```python
from build123d import *

# Parameters (mm, degrees)
SKETCH1_R               = 20.35
BOSS_EXTRUDE2_DEPTH     = 5
SKETCH1_3_R             = 2.35
BOSS_EXTRUDE3_DEPTH     = 10
SKETCH2_R               = 14.85
BOSS_EXTRUDE4_DEPTH     = 7
SKETCH3_R               = 6
SKETCH3_R_2             = 4.1
BOSS_EXTRUDE5_DEPTH     = 10
CUT_EXTRUDE1_DEPTH      = 34.425215033
CUT_EXTRUDE1_DEPTH_BACK = 34.425215033
SKETCH5_R               = 1.6
SKETCH6_R               = 10
CUT_EXTRUDE2_DEPTH      = 9


with BuildPart() as part:
    # Sketch1 → Boss-Extrude2 (new body)
    with BuildSketch(Plane(origin=(0, 0, 0), x_dir=(1, 0, 0), z_dir=(0, 1, 0))):
        with Locations(Location((0, 0, 0), (0, 0, 270))):
            Circle(SKETCH1_R)
    extrude(amount=BOSS_EXTRUDE2_DEPTH)

    # Sketch1_3 → Boss-Extrude3 (add)
    with BuildSketch(Plane(origin=(0, 0, 0), x_dir=(1, 0, 0), z_dir=(0, 1, 0))):
        with Locations(Location((0, 18, 0), (0, 0, 89.999437987))):
            Circle(SKETCH1_3_R)
        with Locations(Location((-17.119017293, 5.562305899, 0), (0, 0, 161.999437549))):
            Circle(SKETCH1_3_R)
        with Locations(Location((-10.580134541, -14.562305899, 0), (0, 0, 233.999434816))):
            Circle(SKETCH1_3_R)
        with Locations(Location((10.580134541, -14.562305899, 0), (0, 0, 305.999433126))):
            Circle(SKETCH1_3_R)
        with Locations(Location((17.119017293, 5.562305899, 0), (0, 0, 17.99943498))):
            Circle(SKETCH1_3_R)
    extrude(amount=BOSS_EXTRUDE3_DEPTH)

    # Sketch2 → Boss-Extrude4 (add)
    with BuildSketch(Plane.XZ):
        with Locations(Location((0, 0, 0), (0, 0, 270))):
            Circle(SKETCH2_R)
    extrude(amount=BOSS_EXTRUDE4_DEPTH)

    # Sketch3 → Boss-Extrude5 (add)
    with BuildSketch(Plane.XZ.offset(7)):
        with Locations(Location((0, 0, 0), (0, 0, 270))):
            Circle(SKETCH3_R)
        with Locations(Location((0, 0, 0), (0, 0, 270))):
            Circle(SKETCH3_R_2, mode=Mode.SUBTRACT)
    extrude(amount=BOSS_EXTRUDE5_DEPTH)

    # Sketch5 → Cut-Extrude1 (cut, two sides: drawn at the far end of the back side and taken through both)
    with BuildSketch(Plane(origin=(0, 0, 0), x_dir=(0, 0, -1), z_dir=(1, 0, 0)).offset(-CUT_EXTRUDE1_DEPTH_BACK)):
        with Locations((0, -11.941738225)):
            Circle(SKETCH5_R)
    extrude(amount=CUT_EXTRUDE1_DEPTH + CUT_EXTRUDE1_DEPTH_BACK, mode=Mode.SUBTRACT)

    # Sketch6 → Cut-Extrude2 (cut)
    with BuildSketch(Plane(origin=(0, 5, 0), x_dir=(1, 0, 0), z_dir=(0, 1, 0))):
        with Locations(Location((0, 0, 0), (0, 0, 270))):
            Circle(SKETCH6_R)
    extrude(amount=-CUT_EXTRUDE2_DEPTH, mode=Mode.SUBTRACT)


solid = part.part
```
The listing builds one solid part. Answer for the finished solid, in the listing's coordinates (mm). A direction names the side the tool comes from. Round coordinates to 2 decimals unless told otherwise and drop trailing zeros. Order: outer loops, then holes, each group sorted by start corner. A loop starts at its lowest first (then second) coordinate and runs counter-clockwise, first axis right, second up. Notation, with made-up numbers: (18.25, 16.5) -> (43.25, 16.5) arc R22 cw to (43.25, 30.5) -> close; hole circle Ø2 at (65.5, 13.5). An arc over 180 degrees is marked (long way). Answer as CSV lines item,"result". Start each with the question number.
(1) The part is cut by section C-C (z = -13). Determine the outline of the cut face in (x, y), then the cut area to 3 significant figures.
(2) Find the intervals of material crossed by probe 1 along X at (y, z) = (-2, 0); probe 2 along Y at (x, z) = (5, 0); probe 3 along X at (y, z) = (0.75, 0), in increasing order. Write a range as from..to.
(3) For a pull along Z with two mould halves and no side action, classify faces 1 (the face through (-9.04, -3.45, 11.78)), 2 (the face through (-4, -17, -3)), 3 (the face through (1.23, -11.93, -3.91)) as +Z half, -Z half, draft (parallel to the pull), parting line (faces both ways), or undercut.
(4) The part is cut by section B-B (y = -9.75). Determine the outline of the cut face in (x, z), then the cut area to 3 significant figures.
(5) The part is cut by section A-A (z = 0). Determine the outline of the cut face in (x, y), then the cut area to 3 significant figures.
(6) A tool of negligible diameter and unlimited length cuts with its end or side. For faces 4 (the face through (-9.72, 7.46, 16.75)), 5 (the face through (-6.4, -7, 0.2)), 6 (the face through (11, 10, 15)), from which of +Z, -Z, +X, -X, +Y, -Y can it reach the whole face along a straight path? Write none if from no direction.
(7) Flat-ended cylindrical pins translate along their axes: pin 1 Ø3.5 at (y, z) = (-11.94, 0) entering from +X; pin 2 Ø4 at (y, z) = (-0.5, 0) entering from -X; pin 3 Ø8 at (x, z) = (-14.5, -13) entering from +Y; pin 4 Ø2 at (x, z) = (-11.5, 11.5) entering from -Y. Find the tip coordinate at first contact, or state that the pin passes through.
(8) The part is cut by section D-D (x = -16.5). Determine the outline of the cut face in (y, z).
Evaluation:
1,outline,"(-15.66, 0) -> (-7.18, 0) -> (-7.18, -7) -> (7.18, -7) -> (7.18, 0) -> (15.66, 0) -> (15.66, 5) -> (-15.66, 5) -> close"
1,area,"257 mm²"
2,probe 1,"-14.85..-10, 10..14.85"
2,probe 2,"-17..-13.54, -10.34..-4"
2,probe 3,"-20.35..-10, 10..20.35"
3,face 1,"parting line"
3,face 2,"draft"
3,face 3,"undercut"
4,outline,"circle Ø12 at (0, 0); hole circle Ø8.2 at (0, 0)"
4,area,"60.3 mm²"
5,outline,"(-20.35, 0) -> (-14.85, 0) -> (-14.85, -7) -> (-6, -7) -> (-6, -10.34) -> (-4.1, -10.34) -> (-4.1, -7) -> (4.1, -7) -> (4.1, -10.34) -> (6, -10.34) -> (6, -7) -> (14.85, -7) -> (14.85, 0) -> (20.35, 0) -> (20.35, 5) -> (10, 5) -> (10, -4) -> (-10, -4) -> (-10, 5) -> (-20.35, 5) -> close; (-6, -17) -> (-4.1, -17) -> (-4.1, -13.54) -> (-6, -13.54) -> close; (4.1, -17) -> (6, -17) -> (6, -13.54) -> (4.1, -13.54) -> close"
5,area,"257 mm²"
6,face 4,"+Y"
6,face 5,"-Y"
6,face 6,"+Z, -Z, +X, -X, +Y"
7,pin 1,"x = 6"
7,pin 2,"x = -20.35"
7,pin 3,"y = 5"
7,pin 4,"y = 0"
8,outline,"(0, -11.91) -> (5, -11.91) -> (5, -7.83) -> (10, -7.83) -> (10, -3.3) -> (5, -3.3) -> (5, 11.91) -> (0, 11.91) -> close"
